Source: CAD feature listing. Evaluate the final solid. Frame: model axes, mm. Face numbers are marked on the shaded views. A direction names the side the tool comes from. Give positions to 0.01 mm unless a question says otherwise; leave off trailing zeros. Order: outer loops, then holes, each group sorted by start corner. A loop starts at its lowest first (then second) coordinate and runs counter-clockwise, first axis right, second up.
from build123d import *

# Parameters (mm, degrees)
SKETCH_3_W          = 457.2
SKETCH_3_H          = 76.2
EXTRUDE_4_DEPTH     = 101.6
SKETCH_3_3_W        = 111.3
SKETCH_3_3_H        = 72.2
SKETCH_3_3_W_2      = 74.2
CUT_EXTRUDE_2_DEPTH = 102.6


with BuildPart() as part:
    # Эскиз3 → Бобышка-Вытянуть4 (new body)
    with BuildSketch(Plane.XY):
        Rectangle(SKETCH_3_W, SKETCH_3_H)
    extrude(amount=EXTRUDE_4_DEPTH)

    # Эскиз3<3> → Вырез-Вытянуть2 (cut, through all)
    with BuildSketch(Plane.XY):
        with Locations((-170.95, 0)):
            Rectangle(SKETCH_3_3_W, SKETCH_3_3_H)
        with Locations((-76.2, 0)):
            Rectangle(SKETCH_3_3_W_2, SKETCH_3_3_H)
        Rectangle(SKETCH_3_3_W_2, SKETCH_3_3_H)
        with Locations((76.2, 0)):
            Rectangle(SKETCH_3_3_W_2, SKETCH_3_3_H)
        with Locations((170.95, 0)):
            Rectangle(SKETCH_3_3_W, SKETCH_3_3_H)
    extrude(amount=CUT_EXTRUDE_2_DEPTH, mode=Mode.SUBTRACT)


solid = part.part
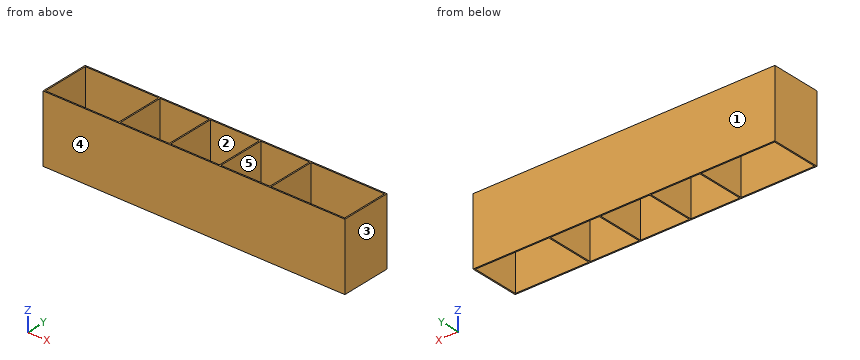
1) Section query A-A on x = -53. Output: boundary loops of the cut face in (y, z), and give its area (3 significant figures).
Checks:
outline: (-38.1, 0) - (-36.1, 0) - (-36.1, 101.6) - (-38.1, 101.6) - close; (36.1, 0) - (38.1, 0) - (38.1, 101.6) - (36.1, 101.6) - close
area: 406 mm2
2) Reachability of the marked faces 1 and 2 from +Z, -Z, +X, -X, +Y, -Y: full face, straight path, thin tool, end or side. Return the list, or none.
Checks:
face 1: +Z, -Z, +X, -X, +Y
face 2: +Z, -Z
3) Section query B-B on y = -7. Output: boundary loops of the cut face in (x, z).
Checks:
outline: (-228.6, 0) - (-226.6, 0) - (-226.6, 101.6) - (-228.6, 101.6) - close; (-115.3, 0) - (-113.3, 0) - (-113.3, 101.6) - (-115.3, 101.6) - close; (-39.1, 0) - (-37.1, 0) - (-37.1, 101.6) - (-39.1, 101.6) - close; (37.1, 0) - (39.1, 0) - (39.1, 101.6) - (37.1, 101.6) - close; (113.3, 0) - (115.3, 0) - (115.3, 101.6) - (113.3, 101.6) - close; (226.6, 0) - (228.6, 0) - (228.6, 101.6) - (226.6, 101.6) - close
4) Section query C-C on z = 38. Output: boundary loops of the cut face in (x, y).
Checks:
outline: (-228.6, -38.1) - (228.6, -38.1) - (228.6, 38.1) - (-228.6, 38.1) - close; hole (-226.6, -36.1) - (-115.3, -36.1) - (-115.3, 36.1) - (-226.6, 36.1) - close; hole (-113.3, -36.1) - (-39.1, -36.1) - (-39.1, 36.1) - (-113.3, 36.1) - close; hole (-37.1, -36.1) - (37.1, -36.1) - (37.1, 36.1) - (-37.1, 36.1) - close; hole (39.1, -36.1) - (113.3, -36.1) - (113.3, 36.1) - (39.1, 36.1) - close; hole (115.3, -36.1) - (226.6, -36.1) - (226.6, 36.1) - (115.3, 36.1) - close
5) Pull-direction query (X, two-part tool) for the marked faces 3, 4 and 5; classes: +X half, -X half, draft (parallel to the pull), parting line (faces both ways), or undercut.
Checks:
face 3: +X half
face 4: draft
face 5: undercut
6) Ray query, L1, parallel to X at y = 5.5, z = 34; L2, parallel to Y at x = -107, z = 55. Return the intervals inside material, ascending.
Checks:
L1: x = -228.6 to -226.6, -115.3 to -113.3, -39.1 to -37.1, 37.1 to 39.1, 113.3 to 115.3, 226.6 to 228.6
L2: y = -38.1 to -36.1, 36.1 to 38.1
